Design review of the part built by this model. Coordinates are the model's own, in mm. A direction names the side the tool comes from. Round coordinates to 2 decimals unless told otherwise and drop trailing zeros. Loops run counter-clockwise (first coordinate to the right, second up) from the corner with the lowest first, then second, coordinate; pieces in that order, holes last. Notation, with made-up numbers: M 86,48 L 131,48 A19 cw 131,63 Z; hole C 10.5,8 d4. An arc over 180 degrees is marked long. One line per item, written item: value. Start each with the question number.
Item 1: For faces 4 (the flat face through (-28, 0, 30)), 5 (the flat face through (0, -3, 28.208)), list the 3-axis set-ups (+Z, -Z, +X, -X, +Y, -Y) from which the entire face can be reached by the end or side of a thin tool; tool diameter is ignored.
Item 2: We need section A-A (x = -62). Write out the cut boundary in (y, z), then the cut area to 3 significant figures.
Item 3: Mouldability with a two-part tool opening along Z and no side actions: class faces 1 (the flat face through (77.352, -3, 32)), 2 (the flat face through (2, -3, 35.115)), 3 (the cylindrical face through (-87.42, -2.5, 23.4)) as released by +Z, released by -Z, zero draft, split by the parting line, or undercut.
Item 4: We need section B-B (z = 33.5). Write out the cut boundary in (x, y), then the cut area to 3 significant figures.
Item 5: Clearance check with a flat-ended pin moving along its axis: pin 1 (3 mm diameter, centred on x = -26.5, y = -1, fed in from -Z). State where the tip first meets the part, or that it passes through.
Item 6: For line 1 along Z through (x, y) = (-49.5, -3.05); line 2 along X through (y, z) = (-2.7, 4.5); line 3 along X through (y, z) = (-2.45, 4), list the stretches that pass through material, from the lowest coordinate up.
from build123d import *

# Parameters (mm, degrees)
F1_DEPTH = 5.08
F2_R     = 5.08


with BuildPart() as f1:
    # F0 (on Front) → F1 (new body)
    with BuildSketch(Plane.XZ):
        with BuildLine():
            Line((77.352171, 35.115106), (-75.047829, 35.115106))
            ThreePointArc((-75.047829, 35.115106), (-94.334729, 27.856756), (-104.050821, 9.683542))
            ThreePointArc((-104.050821, 9.683542), (-98.711588, -2.942531), (-93.372354, 9.683542))
            ThreePointArc((-93.372354, 9.683542), (-88.076021, 22.769908), (-75.047829, 28.207767))
            Line((-75.047829, 28.207767), (77.352171, 28.207767))
            Line((77.352171, 28.207767), (77.352171, 35.115106))
        make_face()
    extrude(amount=F1_DEPTH)

    # F2
    f2_edges = [f1.edges().sort_by_distance(p)[0] for p in [
        (-104.050821, -2.54, 9.683542),
        (-93.372354, -2.54, 9.683542),
        (-75.047829, -2.54, 35.115106),
        (-75.047829, -2.54, 28.207767),
    ]]
    fillet(f2_edges, radius=F2_R)


solid = f1.part
A:
1. face 4: +Z, -Z, +X, -X, +Y
1. face 5: -Z, +X, +Y, -Y
2. outline: M -5.08,28.21 L 0,28.21 L 0,35.12 L -5.08,35.12 Z
2. area: 35.1 mm2
3. face 1: zero draft
3. face 2: released by +Z
3. face 3: undercut
4. outline: M -84.63,-5.08 L 77.35,-5.08 L 77.35,0 L -84.63,0 Z
4. area: 823 mm2
5. pin 1: z = 28.21
6. line 1: 28.21 to 35.12
6. line 2: -106.15 to -91.27
6. line 3: -106.14 to -91.29
